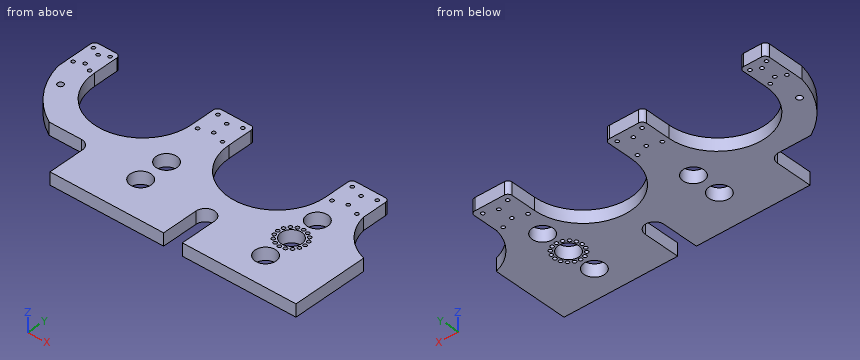
```python
from build123d import *

# Parameters (mm, degrees)
SKETCH1_R           = 25.1
SKETCH1_R_2         = 4.25
SKETCH1_R_3         = 7
BOSS_EXTRUDE1_DEPTH = 30
FILLET1_R           = 10


with BuildPart() as part:
    # Sketch1 → Boss-Extrude1 (new body)
    with BuildSketch(Plane.XY):
        with BuildLine():
            Line((0, 0), (273.87, 0))
            Line((273.87, 0), (273.87, 87.5))
            ThreePointArc((273.87, 87.5), (296.37, 110), (318.87, 87.5))
            Line((318.87, 87.5), (318.87, 0))
            Line((318.87, 0), (592.74, 0))
            Line((592.74, 0), (592.74, 183.19))
            ThreePointArc((592.74, 183.19), (539.268887609, 216.858597344), (511.24, 273.49))
            Line((511.24, 273.49), (511.24, 343.821274963))
            Line((511.24, 343.821274963), (420.37, 343.821274963))
            Line((420.37, 343.821274963), (420.37, 273.49))
            ThreePointArc((420.37, 273.49), (303.87, 156.99), (187.37, 273.49))
            Line((187.37, 273.49), (187.37, 343.821274963))
            Line((187.37, 343.821274963), (96.5, 343.821274963))
            Line((96.5, 343.821274963), (96.5, 273.49))
            ThreePointArc((96.5, 273.49), (-20, 156.99), (-136.5, 273.49))
            Line((-136.5, 273.49), (-136.5, 343.821274963))
            Line((-136.5, 343.821274963), (-199.5, 343.821274963))
            Line((-199.5, 343.821274963), (-199.5, 245.650292451))
            ThreePointArc((-199.5, 245.650292451), (-164.551393078, 166.968268701), (-100, 110))
            Line((-100, 110), (-22.5, 110))
            ThreePointArc((-22.5, 110), (-6.590097423, 103.409902577), (0, 87.5))
            Line((0, 87.5), (0, 0))
        make_face()
        with Locations((455.81, 71.5)):
            Circle(SKETCH1_R, mode=Mode.SUBTRACT)
        with Locations((455.81, 211.5)):
            Circle(SKETCH1_R, mode=Mode.SUBTRACT)
        with Locations((136.93, 91.5)):
            Circle(SKETCH1_R, mode=Mode.SUBTRACT)
        with Locations((136.93, 161.5)):
            Circle(SKETCH1_R, mode=Mode.SUBTRACT)
        with Locations((-188, 328.49)):
            Circle(SKETCH1_R_2, mode=Mode.SUBTRACT)
        with Locations((-188, 273.49)):
            Circle(SKETCH1_R_2, mode=Mode.SUBTRACT)
        with Locations((-148, 328.49)):
            Circle(SKETCH1_R_2, mode=Mode.SUBTRACT)
        with Locations((-148, 273.49)):
            Circle(SKETCH1_R_2, mode=Mode.SUBTRACT)
        with Locations((111.935, 328.49)):
            Circle(SKETCH1_R_2, mode=Mode.SUBTRACT)
        with Locations((171.935, 328.49)):
            Circle(SKETCH1_R_2, mode=Mode.SUBTRACT)
        with Locations((171.935, 273.49)):
            Circle(SKETCH1_R_2, mode=Mode.SUBTRACT)
        with Locations((111.935, 273.49)):
            Circle(SKETCH1_R_2, mode=Mode.SUBTRACT)
        with Locations((495.805, 328.49)):
            Circle(SKETCH1_R_2, mode=Mode.SUBTRACT)
        with Locations((435.805, 328.49)):
            Circle(SKETCH1_R_2, mode=Mode.SUBTRACT)
        with Locations((495.805, 273.49)):
            Circle(SKETCH1_R_2, mode=Mode.SUBTRACT)
        with Locations((435.805, 273.49)):
            Circle(SKETCH1_R_2, mode=Mode.SUBTRACT)
        with Locations((-159.5, 207.5)):
            Circle(SKETCH1_R_3, mode=Mode.SUBTRACT)
        with Locations((-168, 318.49)):
            Circle(SKETCH1_R_2, mode=Mode.SUBTRACT)
        with Locations(Location((-168, 283.49, 0), (0, 0, 180))):
            Circle(SKETCH1_R_2, mode=Mode.SUBTRACT)
        with Locations((141.935, 318.49)):
            Circle(SKETCH1_R_2, mode=Mode.SUBTRACT)
        with Locations(Location((141.935, 283.49, 0), (0, 0, 180))):
            Circle(SKETCH1_R_2, mode=Mode.SUBTRACT)
        with Locations(Location((465.805, 283.49, 0), (0, 0, 180))):
            Circle(SKETCH1_R_2, mode=Mode.SUBTRACT)
        with Locations((465.805, 318.49)):
            Circle(SKETCH1_R_2, mode=Mode.SUBTRACT)
        with Locations((455.81, 141.5)):
            Circle(SKETCH1_R, mode=Mode.SUBTRACT)
        with Locations((455.81, 174.25)):
            Circle(SKETCH1_R_2, mode=Mode.SUBTRACT)
        with Locations((468.34288241, 171.75705469)):
            Circle(SKETCH1_R_2, mode=Mode.SUBTRACT)
        with Locations((478.967747084, 164.657747084)):
            Circle(SKETCH1_R_2, mode=Mode.SUBTRACT)
        with Locations((486.06705469, 154.03288241)):
            Circle(SKETCH1_R_2, mode=Mode.SUBTRACT)
        with Locations((488.56, 141.5)):
            Circle(SKETCH1_R_2, mode=Mode.SUBTRACT)
        with Locations((486.06705469, 128.96711759)):
            Circle(SKETCH1_R_2, mode=Mode.SUBTRACT)
        with Locations((478.967747084, 118.342252916)):
            Circle(SKETCH1_R_2, mode=Mode.SUBTRACT)
        with Locations((468.34288241, 111.24294531)):
            Circle(SKETCH1_R_2, mode=Mode.SUBTRACT)
        with Locations((455.81, 108.75)):
            Circle(SKETCH1_R_2, mode=Mode.SUBTRACT)
        with Locations((443.27711759, 111.24294531)):
            Circle(SKETCH1_R_2, mode=Mode.SUBTRACT)
        with Locations((432.652252916, 118.342252916)):
            Circle(SKETCH1_R_2, mode=Mode.SUBTRACT)
        with Locations((425.55294531, 128.96711759)):
            Circle(SKETCH1_R_2, mode=Mode.SUBTRACT)
        with Locations((423.06, 141.5)):
            Circle(SKETCH1_R_2, mode=Mode.SUBTRACT)
        with Locations((425.55294531, 154.03288241)):
            Circle(SKETCH1_R_2, mode=Mode.SUBTRACT)
        with Locations((432.652252916, 164.657747084)):
            Circle(SKETCH1_R_2, mode=Mode.SUBTRACT)
        with Locations((443.27711759, 171.75705469)):
            Circle(SKETCH1_R_2, mode=Mode.SUBTRACT)
    extrude(amount=BOSS_EXTRUDE1_DEPTH)

    # Fillet1
    fillet1_edges = [part.edges().sort_by_distance(p)[0] for p in [
        (-199.5, 343.821274963, 15),
        (-136.5, 343.821274963, 15),
        (96.5, 343.821274963, 15),
        (187.37, 343.821274963, 15),
        (420.37, 343.821274963, 15),
        (511.24, 343.821274963, 15),
    ]]
    fillet(fillet1_edges, radius=FILLET1_R)


solid = part.part
```
Design review of the part built by this model. Coordinates are the model's own, in mm. Coordinates: 2 decimals unless noted, no trailing zeros. Order: outer loops, then holes, each group sorted by start corner. A loop starts at its lowest first (then second) coordinate and runs counter-clockwise, first axis right, second up. Notation, with made-up numbers: (-28.75, -26.5) - (9.25, -26.5) arc R11 cw to (9.25, -17.5) - close; hole circle Ø6 at (-34, 25). An arc over 180 degrees is marked (long way). Answer in a Markdown table with one row per item.
(1) Wall thickness on line 1 along X through (y, z) = (319, 24.5); line 2 along X through (y, z) = (309.5, 18.5); line 3 along X through (y, z) = (207, 25.5): over which ranges is each line inside the solid? List them lowest first. Write a range as from..to.
Checked values:
| item | result |
|---|---|
| line 1 | -199.5..-172.22, -163.78..-136.5, 96.5..137.72, 146.15..187.37, 420.37..461.59, 470.02..511.24 |
| line 2 | -199.5..-136.5, 96.5..187.37, 420.37..511.24 |
| line 3 | -187.39..-166.48, -152.52..-115.66, 75.66..208.21, 399.53..431.12, 480.5..549.31 |
(2) Consider section C-C on x = 331. State the section outline as (y, z) points, plus the area to 3 significant figures.
Checked values:
| item | result |
|---|---|
| outline | (0, 0) - (160.19, 0) - (160.19, 30) - (0, 30) - close |
| area | 4,810 mm^2 |
(3) Consider section A-A on x = 52. State the section outline as (y, z) points, plus the area to 3 significant figures.
Checked values:
| item | result |
|---|---|
| outline | (0, 0) - (181.9, 0) - (181.9, 30) - (0, 30) - close |
| area | 5,460 mm^2 |
(4) Consider section B-B on z = 7. Give the number of separate pieces and of enclosed holes in the cut face, plus the area to 3 significant figures.
Checked values:
| item | result |
|---|---|
| separate pieces | 1 |
| enclosed holes | 40 |
| area | 143,000 mm^2 |
(5) Clearance check with flat-ended pins moving along their axes: pin 1 (12 mm diameter, centred on x = -53, z = 26.5, fed in from +Y); pin 2 (10 mm diameter, centred on x = -57.5, z = 3, fed in from +Y); pin 3 (5 mm diameter, centred on x = 171.935, y = 273.49, fed in from -Z); pin 4 (15 mm diameter, centred on y = 311, z = 15.5, fed in from +X). State where each tip first meets the part, or that it passes through.
Checked values:
| item | result |
|---|---|
| pin 1 | y = 163.71 |
| pin 2 | y = 165.02 |
| pin 3 | through |
| pin 4 | x = 511.24 |
